The listing builds one solid part. Answer for the finished solid, in the listing's coordinates (mm). A direction names the side the tool comes from. Round coordinates to 2 decimals unless told otherwise and drop trailing zeros. Order: outer loops, then holes, each group sorted by start corner. A loop starts at its lowest first (then second) coordinate and runs counter-clockwise, first axis right, second up. Notation, with made-up numbers: M 68.5,-28 L 118.5,-28 A25 ccw 118.5,-13 Z; hole C 28.25,28.5 d2. An arc over 180 degrees is marked long. Write item = value, one per line. Start each with the question number.
(1) A cutting plane is placed at B-B, the plane x = 0. Determine the outline of the cut face in (y, z) (3 decimals), and give its area (3 significant figures).
(2) For a pull along X with two mould halves and no side action, classify faces 5 (the face through (-18.21, -10.46, 30.45)), 6 (the face through (-7, 18, 65)), 7 (the face through (8.87, 17.64, 30.45)), 8 (the face through (-3, 0, -10.05)) as released by +X, released by -X, zero draft, split by the parting line, or undercut.
(3) Straight lines are drawn through the part: probe 1 along X at (y, z) = (0, -2.2); probe 2 along Y at (x, z) = (0, -7.25); probe 3 along Y at (x, z) = (0, -3). For each, find the intervals that lie inside material, in ascending order. Write a range as from..to.
(4) Which of the six approach directions +Z, -Z, +X, -X, +Y, -Y give full straight-line access (tool end or side, diameter ignored) to faces 1 (the face through (13.9, 7.92, 35.49)), 2 (the face through (-7.73, 18.3, 30.45)), 3 (the face through (-14.735, -8.478, 48.025)), 4 (the face through (-11, 6.2, -10.7))?
(5) A cutting plane is placed at A-A, the plane z = 23.5. Determine the outline of the cut face in (x, y).
(6) Each of these flat-tipped pins is pushed along its axis until it touches: pin 1 (2 mm diameter, centred on y = 13, z = 54.5, fed in from -X); pin 2 (6 mm diameter, centred on x = -4, z = 34, fed in from -Y); pin 3 (3 mm diameter, centred on x = -14.5, y = 16.5, fed in from -Z); pin 4 (4 mm diameter, centred on x = 12.5, z = 46.5, fed in from +Y). Where does it stop, or does it pass through?
from build123d import *

# Parameters (mm, degrees)
SKETCH2_R               = 16
BOSS_EXTRUDE1_DEPTH     = 82.25
CUT_EXTRUDE1_DEPTH      = 97.457244414
CUT_EXTRUDE1_DEPTH_BACK = 97.457244414
SKETCH3_W               = 152.01959988
SKETCH3_H               = 124.433031562
CUT_EXTRUDE2_DEPTH      = 1.7
CHAMFER2_SIZE           = 1
CHAMFER3_SIZE           = 1
CUT_EXTRUDE3_DEPTH      = 71
CHAMFER4_SIZE           = 1
CUT_EXTRUDE4_DEPTH      = 1.2
SKETCH8_R               = 2.75
CUT_EXTRUDE5_DEPTH      = 87.332400234
CUT_EXTRUDE7_DEPTH      = 5
CHAMFER5_SIZE           = 0.5
CUT_EXTRUDE8_DEPTH      = 88.459952722
SKETCH12_R              = 1.8
CUT_EXTRUDE9_DEPTH      = 4
CUT_EXTRUDE10_START     = -4
SKETCH13_R              = 1.8
CUT_EXTRUDE10_DEPTH     = 4


with BuildPart() as part:
    # Sketch1 → Revolve1 (revolve)
    with BuildSketch(Plane(origin=(0, 0, 0), x_dir=(1, 0, 0), z_dir=(0, 1, 0))):
        Polygon((0, 0), (16.125, 0), (16.125, -71), (19.65, -71), (19.65, 68), (24.95, 68), (24.95, 73), (28.1, 73), (28.1, 68), (42, 68), (42, 76), (16.65, 76), (16.65, 18.004366875), (12.193967069, 18.004366875), (12.193967069, 24.882682167), (0, 24.882682167), align=None)
    revolve(axis=Axis((0, 0, 39.840023079), (0, 0, -1)))

    # Sketch2 → Boss-Extrude1 (add)
    with BuildSketch(Plane.XY.offset(71)):
        Polygon((0, 22.762034363), (-19.7125, 11.381017181), (-19.7125, -11.381017181), (0, -22.762034363), (19.7125, -11.381017181), (19.7125, 11.381017181), align=None)
        Circle(SKETCH2_R, mode=Mode.SUBTRACT)
    extrude(amount=-BOSS_EXTRUDE1_DEPTH)

    # Sketch3 → Cut-Extrude1 (cut, two sides: drawn at the far end of the back side and taken through both)
    with BuildSketch(Plane(origin=(0, 0, 0), x_dir=(1, 0, 0), z_dir=(0, 1, 0)).offset(-CUT_EXTRUDE1_DEPTH_BACK)):
        with Locations((6.162956752, 73.466515781)):
            Rectangle(SKETCH3_W, SKETCH3_H)
    extrude(amount=CUT_EXTRUDE1_DEPTH + CUT_EXTRUDE1_DEPTH_BACK, mode=Mode.SUBTRACT)

    # Sketch4 → Cut-Extrude2 (cut)
    with BuildSketch(Plane(origin=(-9.85625, 17.071525772, 0), x_dir=(0.8660254037844386, 0.5000000000000003, 0), z_dir=(-0.5000000000000002, 0.8660254037844385, 0))):
        Polygon((-8.6, 10.2), (4.6, 10.2), (4.6, 5.2), (1.6, 5.2), (1.6, -65), (4.6, -65), (4.6, -70), (-8.6, -70), align=None)
    extrude(amount=-CUT_EXTRUDE2_DEPTH, mode=Mode.SUBTRACT)

    # Chamfer2
    chamfer2_edges = [part.edges().sort_by_distance(p)[0] for p in [
        (0, 22.762034363, 29.875),
        (19.7125, 11.381017181, 29.875),
        (19.7125, -11.381017181, 29.875),
        (0, -22.762034363, 29.875),
        (-19.7125, -11.381017181, 29.875),
        (-19.7125, 11.381017181, 29.875),
    ]]
    chamfer(chamfer2_edges, length=CHAMFER2_SIZE)

    # Chamfer3
    chamfer3_edges = [part.edges().sort_by_distance(p)[0] for p in [
        (-16, 0, 71),
    ]]
    chamfer(chamfer3_edges, length=CHAMFER3_SIZE)

    # Sketch5 → Cut-Extrude3 (cut)
    with BuildSketch(Plane.XY.offset(71)):
        with BuildLine():
            Line((-17, 9.814954576), (-15.92887426, -1.50697207))
            ThreePointArc((-15.92887426, -1.50697207), (-8, 13.85640646), (9.269513225, 13.041323728))
            Line((9.269513225, 13.041323728), (0, 19.629909152))
            Line((0, 19.629909152), (-17, 9.814954576))
        make_face()
        with BuildLine():
            Line((0, -19.629909152), (17, -9.814954576))
            Line((17, -9.814954576), (15.92887426, 1.50697207))
            ThreePointArc((15.92887426, 1.50697207), (8, -13.856406461), (-9.269513225, -13.041323728))
            Line((-9.269513225, -13.041323728), (0, -19.629909152))
        make_face()
    extrude(amount=-CUT_EXTRUDE3_DEPTH, mode=Mode.SUBTRACT)

    # Chamfer4
    chamfer4_edges = [part.edges().sort_by_distance(p)[0] for p in [
        (0, -19.629909152, 35.5),
        (17, -9.814954576, 35.5),
        (0, 19.629909152, 35.5),
        (-17, 9.814954576, 35.5),
    ]]
    chamfer(chamfer4_edges, length=CHAMFER4_SIZE)

    # Sketch6 → Cut-Extrude4 (cut)
    with BuildSketch(Plane(origin=(0, 0, -11.25), x_dir=(-1, 0, 0), z_dir=(0, 0, -1))):
        Polygon((-7.289047149, 12.625), (-14.578094297, 0), (-7.289047149, -12.625), (7.289047149, -12.625), (14.578094297, 0), (7.289047149, 12.625), align=None)
    extrude(amount=-CUT_EXTRUDE4_DEPTH, mode=Mode.SUBTRACT)

    # Sketch8 → Cut-Extrude5 (cut, through all)
    with BuildSketch(Plane(origin=(0, 0, -10.05), x_dir=(-1, 0, 0), z_dir=(0, 0, -1))):
        Circle(SKETCH8_R)
    extrude(amount=-CUT_EXTRUDE5_DEPTH, mode=Mode.SUBTRACT)

    # Sketch10 → Cut-Extrude7 (cut)
    with BuildSketch(Plane.XY):
        with BuildLine():
            Line((2.5, 10), (-2.5, 10))
            Line((-2.5, 10), (-2.5, 7.071067812))
            ThreePointArc((-2.5, 7.071067812), (0, -7.5), (2.5, 7.071067812))
            Line((2.5, 7.071067812), (2.5, 10))
        make_face()
    extrude(amount=-CUT_EXTRUDE7_DEPTH, mode=Mode.SUBTRACT)

    # Chamfer5
    chamfer5_edges = [part.edges().sort_by_distance(p)[0] for p in [
        (0, -7.5, 0),
        (2.5, 8.535533906, 0),
        (0, 10, 0),
        (-2.5, 8.535533906, 0),
    ]]
    chamfer(chamfer5_edges, length=CHAMFER5_SIZE)

    # Sketch11 → Cut-Extrude8 (cut, through all)
    with BuildSketch(Plane.XY.offset(71)):
        Polygon((19.7125, 11.381017181), (16.660566959, 13.143051544), (19.7125, 7.856948456), align=None)
        Polygon((-16.660566959, -13.143051544), (-19.7125, -11.381017181), (-19.7125, -7.856948456), align=None)
    extrude(amount=-CUT_EXTRUDE8_DEPTH, mode=Mode.SUBTRACT)

    # Sketch12 → Cut-Extrude9 (cut)
    with BuildSketch(Plane(origin=(-18.186533479, -10.5, 0), x_dir=(0, 0, 1), z_dir=(-0.8660254037844382, -0.500000000000001, 0))):
        with Locations(Location((48, 0, 0), (0, 0, 270))):
            Circle(SKETCH12_R)
    extrude(amount=-CUT_EXTRUDE9_DEPTH, mode=Mode.SUBTRACT)

    # Sketch13 → Cut-Extrude10 (cut)
    with BuildSketch(Plane(origin=(18.186533479, 10.5, 0), x_dir=(0, 0, -1), z_dir=(0.8660254037844387, 0.4999999999999999, 0)).offset(CUT_EXTRUDE10_START)):
        with Locations(Location((-48, 0, 0), (0, 0, 270))):
            Circle(SKETCH13_R)
    extrude(amount=CUT_EXTRUDE10_DEPTH, mode=Mode.SUBTRACT)


solid = part.part
Reported:
q1.outline = M -22.262,-11.25 L -12.625,-11.25 L -12.625,-10.05 L -2.75,-10.05 L -2.75,-5 L -7.5,-5 L -7.5,-0.5 L -8,0 L -19.089,0 L -19.089,71 L -22.262,71 Z; M 2.75,-10.05 L 12.625,-10.05 L 12.625,-11.25 L 22.262,-11.25 L 22.262,71 L 19.089,71 L 19.089,0 L 10.5,0 L 10,-0.5 L 10,-5 L 2.75,-5 Z
q1.area = 806 mm²
q2.face_5 = released by -X
q2.face_6 = zero draft
q2.face_7 = released by +X
q2.face_8 = undercut
q3.probe_1 = -19.71..-7.5, 7.5..19.71
q3.probe_2 = -22.26..-2.75, 2.75..22.26
q3.probe_3 = -22.26..-7.5, 10..22.26
q4.face_1 = +Z
q4.face_2 = +Z, -Z, -X, +Y
q4.face_3 = none
q4.face_4 = -Z
q5.outline = M -19.71,-7.86 L -16.66,-13.14 L -0.87,-22.26 L 0.87,-22.26 L 18.85,-11.88 L 19.71,-10.38 L 19.71,7.86 L 16.66,13.14 L 0.87,22.26 L -0.87,22.26 L -8.47,17.87 L -7.62,16.4 L -16.45,11.3 L -17.3,12.77 L -18.85,11.88 L -19.71,10.38 Z; hole M -16.91,8.82 L -15.93,-1.51 A16 ccw -9.27,-13.04 L -0.82,-19.05 L 0.87,-19.13 L 16.13,-10.31 L 16.91,-8.82 L 15.93,1.51 A16 ccw 9.27,13.04 L 0.82,19.05 L -0.87,19.13 L -16.13,10.31 Z
q6.pin_1 = -18.64
q6.pin_2 = -22.18
q6.pin_3 = through
q6.pin_4 = 16.7
